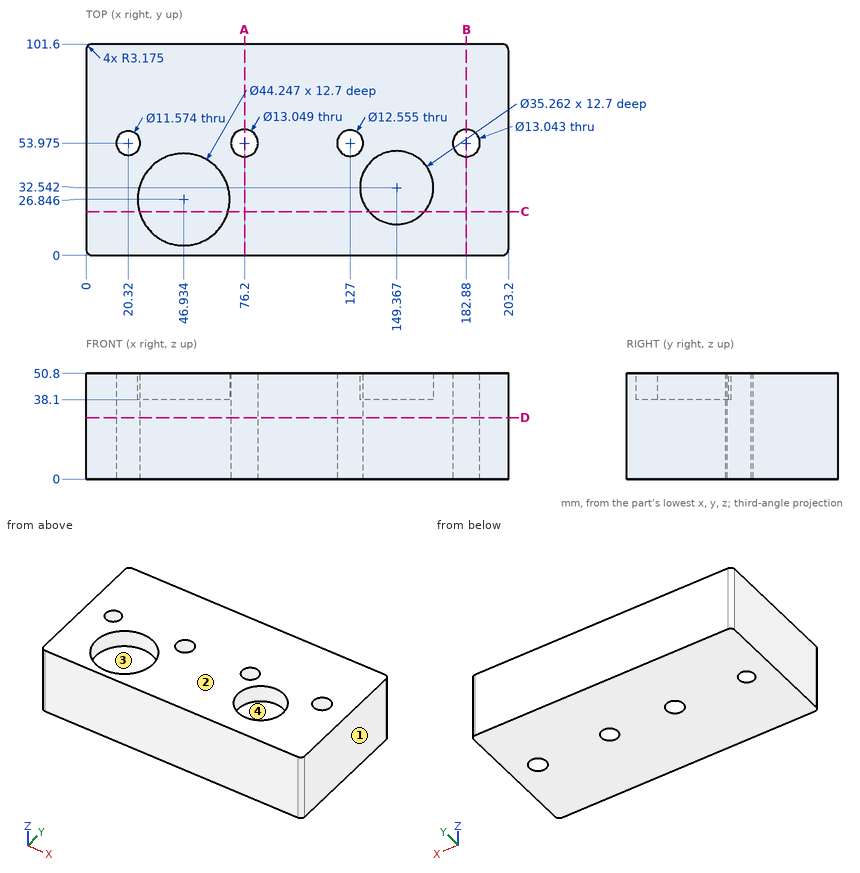
Verification items for this drawing (mm, ordinates from the low corner). Give positions to 0.01 mm unless a question says otherwise; leave off trailing zeros. Loops run counter-clockwise (first coordinate to the right, second up) from the corner with the lowest first, then second, coordinate; pieces in that order, holes last. Notation, with made-up numbers: (-40, -31) - (18, -31) arc R35 cw to (18, 7) - close; hole circle Ø1 at (63, 39.25). An arc over 180 degrees is marked (long way). Write item = value, one per line. Start each with the question number.
Q1. Cross-section at C-C, the plane y = 21. Enter the section's corners in (x, z) (1 decimal), and give its area (3 significant figures).
Q2. Thickness scan on line 1 (Y direction, x = 182.88, z = 16); line 2 (Y direction, x = 20, z = 18); line 3 (Z direction, x = 52, y = 21). Record the ranges inside material, lowest first.
Q3. Mould release check, pull along X, two halves, no side actions. Record for the marked faces 1, 2, 3 and 4: released by +X, released by -X, zero draft, split by the parting line, or undercut.
Q4. Depth check by flat-ended pin: P1, Ø10.5, axis at x = 76.2, y = 53.975, coming from the -Z side; P2, Ø10.5, axis at x = 157, y = 33.5, coming from the +Z side. Enter the tip coordinate at first touch or a pass-through.
Q5. Cross-section at D-D, the plane z = 29.5. State how many separate pieces and enclosed holes the cut face has, and give its area (3 significant figures).
Q6. Cross-section at A-A, the plane x = 76.2. Enter the section's corners in (y, z).
Answer key:
q1.outline = (0, 0) - (203.2, 0) - (203.2, 50.8) - (162.7, 50.8) - (162.7, 38.1) - (136, 38.1) - (136, 50.8) - (68.3, 50.8) - (68.3, 38.1) - (25.6, 38.1) - (25.6, 50.8) - (0, 50.8) - close
q1.area = 9,440 mm^2
q2.line_1 = 0 to 47.45, 60.5 to 101.6
q2.line_2 = 0 to 48.2, 59.75 to 101.6
q2.line_3 = 0 to 38.1
q3.face_1 = released by +X
q3.face_2 = zero draft
q3.face_3 = undercut
q3.face_4 = undercut
q4.P1 = through
q4.P2 = 38.1
q5.separate_pieces = 1
q5.enclosed_holes = 4
q5.area = 20,100 mm^2
q6.outline = (0, 0) - (47.45, 0) - (47.45, 50.8) - (0, 50.8) - close; (60.5, 0) - (101.6, 0) - (101.6, 50.8) - (60.5, 50.8) - close
